Design review of the part built by this model. Coordinates are the model's own, in mm. Round coordinates to 2 decimals unless told otherwise and drop trailing zeros. Loops run counter-clockwise (first coordinate to the right, second up) from the corner with the lowest first, then second, coordinate; pieces in that order, holes last. Notation, with made-up numbers: (15, -29.75) -> (68, -29.75) arc R35 ccw to (68, 9.25) -> close; hole circle Ø7 at (-39.5, 37). An arc over 180 degrees is marked (long way). Answer as CSV lines item,"result". Start each with the question number.
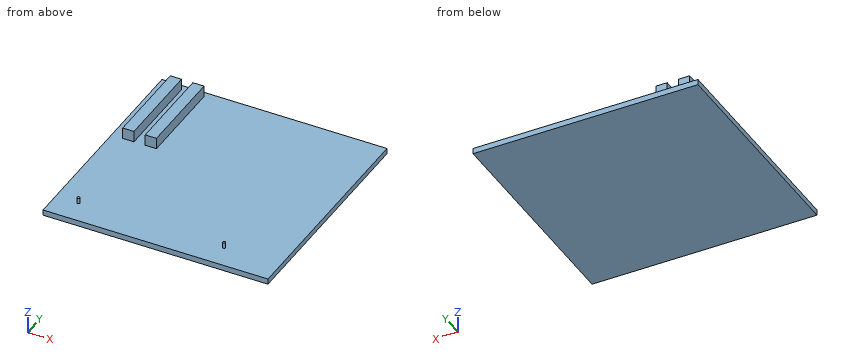
Autodesk Inventor part; units mm, degrees
ref_plane "YZ Plane" through (0, 0, 0) normal (1, 0, 0) x (0, 1, 0)
ref_plane "XZ Plane" through (0, 0, 0) normal (0, 1, 0) x (-1, 0, 0)
ref_plane "XY Plane" through (0, 0, 0) normal (0, 0, 1) x (1, 0, 0)
sketch "Sketch1" plane through (0, 0, 0) normal (0, 0, 1) x (1, 0, 0)
  line L0 (0, 0) -> (508, 0)
  line L1 (508, 0) -> (508, 508)
  line L2 (508, 508) -> (0, 508)
  line L3 (0, 508) -> (0, 0)
  dimension "d0" = 508
  dimension "d1" = 508
extrude "Extrusion1" add sketch "Sketch1" along normal blind 12.7
sketch "Sketch2" plane through (0, 0, 12.7) normal (0, 0, 1) x (1, 0, 0)
  circle A0 centre (51.0764, 55.0392) radius 3.175
  circle A1 centre (379.8659, 55.0392) radius 3.175
  point P0 (0, 0)
  dimension "d4" = 6.35
  dimension "d5" = 6.35
extrude "Extrusion2" add sketch "Sketch2" along normal blind 12.7
sketch "Sketch3" plane through (0, 0, 12.7) normal (0, 0, 1) x (1, 0, 0)
  line L0 (25.4, 495.3) -> (50.8, 495.3)
  line L1 (50.8, 495.3) -> (50.8, 292.1)
  line L2 (50.8, 292.1) -> (25.4, 292.1)
  line L3 (25.4, 292.1) -> (25.4, 495.3)
  line L4 (76.2, 495.3) -> (101.6, 495.3)
  line L5 (101.6, 495.3) -> (101.6, 292.1)
  line L6 (101.6, 292.1) -> (76.2, 292.1)
  line L7 (76.2, 292.1) -> (76.2, 495.3)
  line L8 (508, 508) -> (0, 508)
  line L9 (0, 508) -> (0, 0)
  dimension "d8" = 25.4
  dimension "d9" = 203.2
  dimension "d10" = 25.4
  dimension "d11" = 203.2
  dimension "d12" = 25.4
  dimension "d15" = 12.7
  dimension "d16" = 12.7
  dimension "d17" = 50.8
extrude "Extrusion3" add sketch "Sketch3" along normal blind 25.4
properties part number "Base"
Q1. Add section B-B, the plane x = 339. Give the boundary of the cut face in (y, z).
Q2. Add section A-A, the plane y = 447.5. Give the boundary of the cut face in (x, z).
Q3. For pin 1 Ø1.5 at (x, y) = (188, 345) entering from +Z; pin 2 Ø12.5 at (y, z) = (381, 27) entering from -X; pin 3 Ø5 at (x, y) = (378.5, 55.5) entering from +Z, all flat-tipped, find the tip position at first contact; note any pin that passes through.
Q4. To check wall thickness, follow probe 1 along X at (y, z) = (403, 15); probe 2 along Z at (x, y) = (339, 345.5); probe 3 along Y at (x, z) = (84.5, 28). State the ranges of each line that lie inside material, in increasing order. Write a range as from..to.
Worked answers:
1,outline,"(0, 0) -> (508, 0) -> (508, 12.7) -> (0, 12.7) -> close"
2,outline,"(0, 0) -> (508, 0) -> (508, 12.7) -> (101.6, 12.7) -> (101.6, 38.1) -> (76.2, 38.1) -> (76.2, 12.7) -> (50.8, 12.7) -> (50.8, 38.1) -> (25.4, 38.1) -> (25.4, 12.7) -> (0, 12.7) -> close"
3,pin 1,"stops at z = 12.7"
3,pin 2,"stops at x = 25.4"
3,pin 3,"stops at z = 25.4"
4,probe 1,"x = 25.4..50.8, 76.2..101.6"
4,probe 2,"z = 0..12.7"
4,probe 3,"y = 292.1..495.3"
